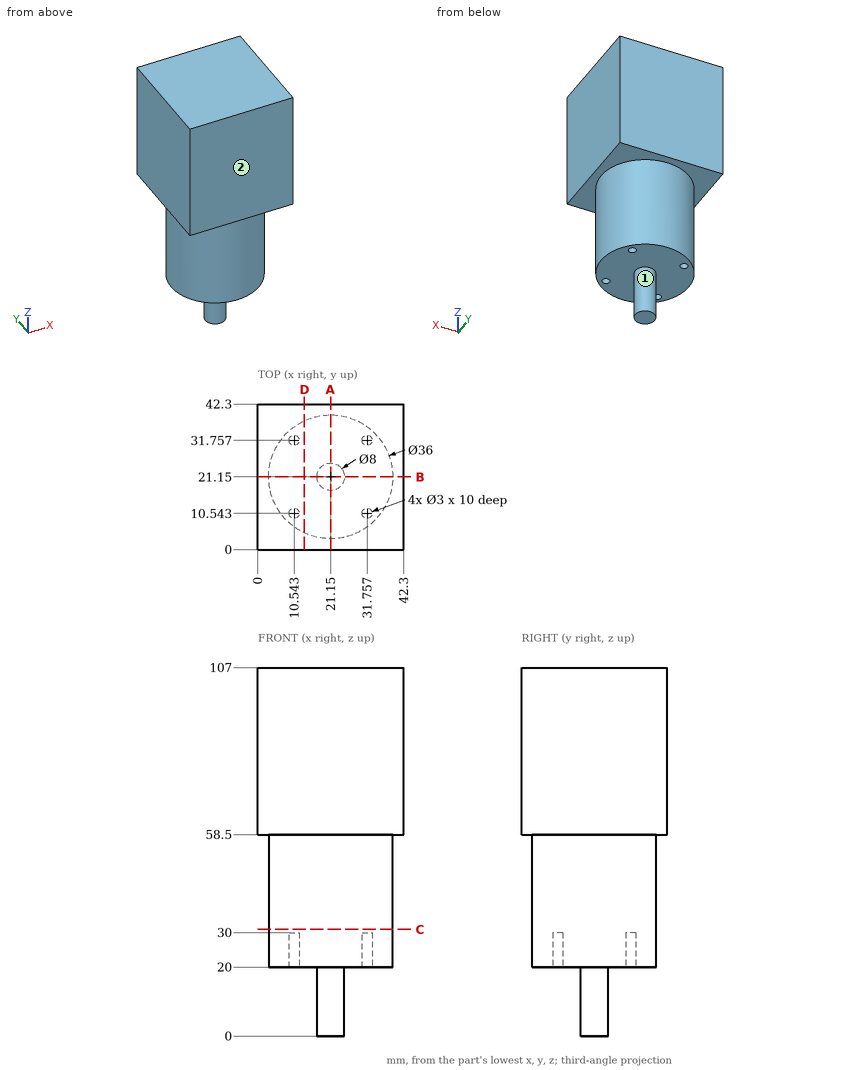
Design review of the part shown in the three views and the two pictorial views. Dimensions are in mm from the part's minimum x, y and z. A direction names the side the tool comes from. Give positions to 0.01 mm unless a question says otherwise; leave off trailing zeros. Loops run counter-clockwise (first coordinate to the right, second up) from the corner with the lowest first, then second, coordinate; pieces in that order, holes last. Notation, with made-up numbers: M 13.5,55.25 L 31.5,55.25 A21 cw 31.5,76.25 Z; hole C 30,46 d7. An arc over 180 degrees is marked long. Write item = value, one per line.
Q1. For the marked faces 1 and 2, list the 3-axis set-ups (+Z, -Z, +X, -X, +Y, -Y) from which the entire face can be reached by the end or side of a thin tool; tool diameter is ignored.
Output values:
face_1 = -Z
face_2 = +Z, -Z, +X, -X, -Y
Q2. Insertion check: pin 1 (4 mm diameter, centred on x = 15.5, z = 30.5, fed in from -Y); pin 2 (3.5 mm diameter, centred on x = 11, y = 31.5, fed in from -Z); pin 3 (3 mm diameter, centred on y = 17, z = 48, fed in from -X). Each pin has a flat end and moves straight along its axis. Give the tip position at first contact, or say it passes through.
Output values:
pin_1 = 3.52
pin_2 = 20
pin_3 = 3.35
Q3. We need section A-A (x = 21.15). Give the boundary of the cut face in (y, z).
Output values:
outline = M 0,58.5 L 3.15,58.5 L 3.15,20 L 17.15,20 L 17.15,0 L 25.15,0 L 25.15,20 L 39.15,20 L 39.15,58.5 L 42.3,58.5 L 42.3,107 L 0,107 Z
Q4. We need section C-C (z = 31). Give the boundary of the cut face in (x, y).
Output values:
outline = C 21.15,21.15 d36
Q5. We need section D-D (x = 13.5). Give the boundary of the cut face in (y, z), plus the area to 3 significant figures.
Output values:
outline = M 0,58.5 L 4.86,58.5 L 4.86,20 L 37.44,20 L 37.44,58.5 L 42.3,58.5 L 42.3,107 L 0,107 Z
area = 3,310 mm^2
Q6. To check wall thickness, follow line 1 (Y direction, x = 21, z = 43); line 2 (Z direction, x = 37, y = 36); line 3 (Z direction, x = 18, y = 34). State the ranges of each line that lie inside material, in increasing order. Write a range as [from, to].
Output values:
line_1 = [3.15, 39.15]
line_2 = [58.5, 107]
line_3 = [20, 107]
